Design review of the part shown in the three views and the two pictorial views. Dimensions are in mm from the part's minimum x, y and z. Round coordinates to 2 decimals unless told otherwise and drop trailing zeros. Loops run counter-clockwise (first coordinate to the right, second up) from the corner with the lowest first, then second, coordinate; pieces in that order, holes last.
1. Clearance check with flat-ended pins moving along their axes: pin 1 Ø3 at (x, z) = (3, 3.5) entering from +Y; pin 2 Ø8 at (x, y) = (8.5, 29.5) entering from -Z. State where each tip first meets the part, or that it passes through.
2. Consider section D-D on x = 6. State the section outline as (y, z) points.
3. Consider section C-C on z = 2.8. State the section outline as (x, y) points.
4. Consider section B-B on y = 8. State the section outline as (x, z) points, then the cut area to 3 significant figures.
5. To check wall thickness, follow line 1 along Y through (x, z) = (8, 4.9); line 2 along X through (y, z) = (30, 5.75); line 3 along Y through (x, z) = (10.75, 3.8). State the ranges of each line that lie inside material, in increasing order.
6. Draft analysis for pull direction Y (two halves, no side actions). For the marked faces 1, 2 and 3, state which applies: released by +Y, released by -Y, zero draft, split by the parting line, or undercut.
7. Consider section A-A on x = 7.5. State the section outline as (y, z) points, then the cut area to 3 significant figures.
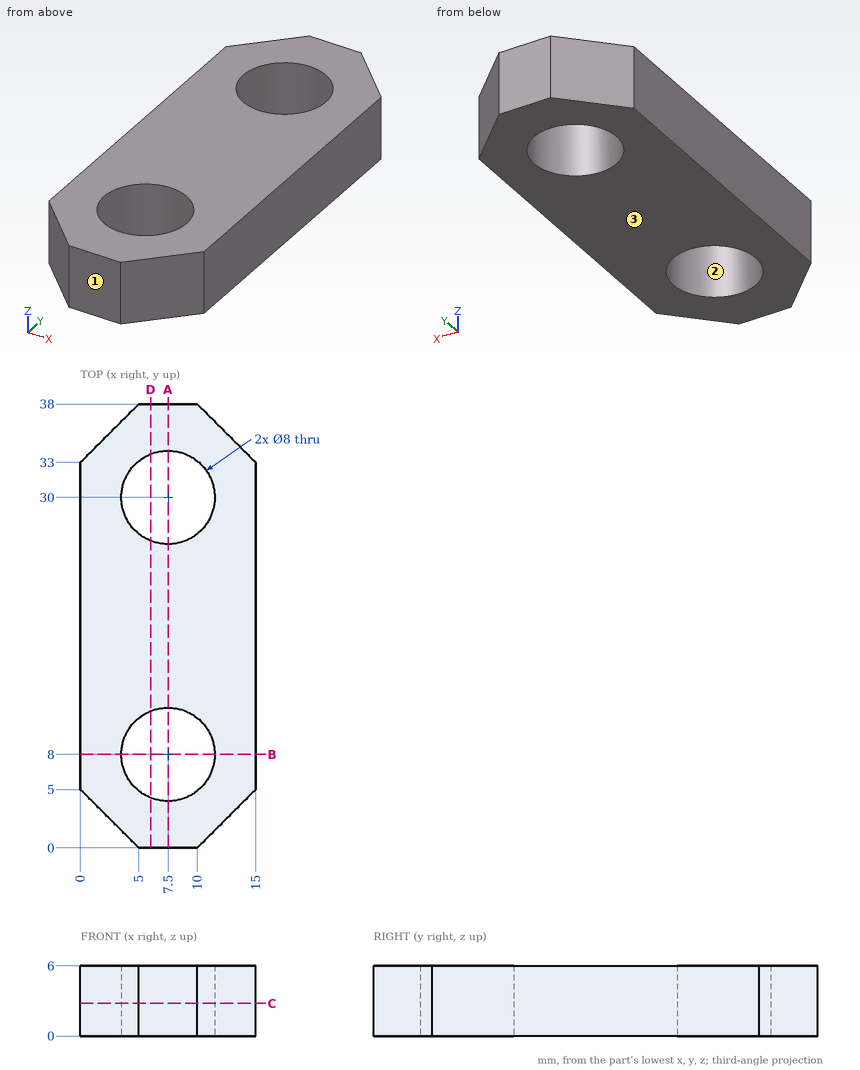
Resolved:
1. pin 1: stops at y = 37.5
1. pin 2: stops at z = 0
2. outline: (0, 0) - (4.29, 0) - (4.29, 6) - (0, 6) - close; (11.71, 0) - (26.29, 0) - (26.29, 6) - (11.71, 6) - close; (33.71, 0) - (38, 0) - (38, 6) - (33.71, 6) - close
3. outline: (0, 5) - (5, 0) - (10, 0) - (15, 5) - (15, 33) - (10, 38) - (5, 38) - (0, 33) - close; hole circle Ø8 at (7.5, 8); hole circle Ø8 at (7.5, 30)
4. outline: (0, 0) - (3.5, 0) - (3.5, 6) - (0, 6) - close; (11.5, 0) - (15, 0) - (15, 6) - (11.5, 6) - close
4. area: 42.0 mm2
5. line 1: y = 0 to 4.03, 11.97 to 26.03, 33.97 to 38
5. line 2: x = 0 to 3.5, 11.5 to 15
5. line 3: y = 0.75 to 5.67, 10.33 to 27.67, 32.33 to 37.25
6. face 1: released by -Y
6. face 2: undercut
6. face 3: zero draft
7. outline: (0, 0) - (4, 0) - (4, 6) - (0, 6) - close; (12, 0) - (26, 0) - (26, 6) - (12, 6) - close; (34, 0) - (38, 0) - (38, 6) - (34, 6) - close
7. area: 132 mm2
